```python
from build123d import *

# Parameters (mm, degrees)
PAD_DEPTH       = 9
SKETCH001_R     = 1.5
POCKET_DEPTH    = 13.501
SKETCH002_R     = 3
POCKET001_DEPTH = 11
PAD001_DEPTH    = 2
POCKET002_DEPTH = 2.501


with BuildPart() as part:
    # Sketch → Pad (new body)
    with BuildSketch(Plane.XY):
        with BuildLine():
            Line((-7, -4), (-31, -4))
            Line((-31, -4), (-31, -6.5))
            Line((-31, -6.5), (16, -6.5))
            Line((16, -6.5), (16, -3.5))
            Line((16, -3.5), (1.936492, -3.5))
            ThreePointArc((1.936492, 3.5), (-4, 0), (1.936492, -3.5))
            Line((1.936492, 3.5), (16, 3.5))
            Line((16, 7), (16, 3.5))
            Line((0, 7), (16, 7))
            Line((-7, 7), (0, 7))
            Line((-7, -4), (-7, 7))
        make_face()
    extrude(amount=PAD_DEPTH)

    # Sketch001 → Pocket (cut, through all)
    with BuildSketch(Plane.XZ.offset(6.5)):
        with Locations((-27.5, 4.5)):
            Circle(SKETCH001_R)
        with Locations((-8.5, 4.5)):
            Circle(SKETCH001_R)
        with Locations((10.5, 4.5)):
            Circle(SKETCH001_R)
    extrude(amount=-POCKET_DEPTH, mode=Mode.SUBTRACT)

    # Sketch002 → Pocket001 (cut)
    with BuildSketch(Plane(origin=(0, 7, 0), x_dir=(-1, 0, 0), z_dir=(0, 1, 0))):
        with Locations((8.5, 4.5)):
            Circle(SKETCH002_R)
    extrude(amount=-POCKET001_DEPTH, mode=Mode.SUBTRACT)

    # Sketch003 → Pad001 (new body)
    with BuildSketch(Plane(origin=(0, 7, 0), x_dir=(-1, 0, 0), z_dir=(0, 1, 0))):
        Polygon((-13.098076, 9), (-15.696152, 4.5), (-13.098076, 0), (-7.901924, 0), (-5.303848, 4.5), (-7.901924, 9), align=None)
        Polygon((-9, 1.901924), (-7.5, 4.5), (-9, 7.098076), (-12, 7.098076), (-13.5, 4.5), (-12, 1.901924), align=None, mode=Mode.SUBTRACT)
    extrude(amount=PAD001_DEPTH)

    # Sketch004 → Pocket002 (cut, through all)
    with BuildSketch(Plane(origin=(0, -4, 0), x_dir=(-1, 0, 0), z_dir=(0, 1, 0))):
        Polygon((31, 6), (28, 9), (31, 9), align=None)
        Polygon((28, 0), (31, 0), (31, 3), align=None)
    extrude(amount=-POCKET002_DEPTH, mode=Mode.SUBTRACT)


solid = part.part
```
Work out the finished part from the listing and answer in its coordinate system (mm). A direction names the side the tool comes from. Give positions to 0.01 mm unless a question says otherwise; leave off trailing zeros. Write each loop counter-clockwise with the first axis right and the second up, starting at its lowest first coordinate (ties: lowest second). Pieces come first, ordered by that corner, then holes. Notation, with made-up numbers: (50.25, -5.75) -> (91.25, -5.75) arc R32 ccw to (91.25, 31.25) -> close; hole circle Ø10 at (63, -17). An arc over 180 degrees is marked (long way). Write item = value, one per line.
Q1. Section B-B on x = 0 is taken. Determine the outline of the cut face in (y, z), and give its area (3 significant figures).
Computed values:
outline = (-6.5, 0) -> (-4, 0) -> (-4, 9) -> (-6.5, 9) -> close; (4, 0) -> (7, 0) -> (7, 9) -> (4, 9) -> close
area = 49.5 mm^2
Q2. A tool of negligible diameter and unlimited length cuts with its end or side. For faces 5 (the flat face through (14.415, 7.986, 2.281)), 6 (the flat face through (6.62, 7.99, 2.22)), 7 (the flat face through (-7, 1, 1)), 8 (the flat face through (8.24, 7.99, 5.78)), 9 (the flat face through (15.5, 7, 3.4)), from which of +Z, -Z, +X, -X, +Y, -Y can it reach the whole face along a straight path? Write none if from no direction.
Computed values:
face_5 = -Z, +X, +Y
face_6 = -Z, -X, +Y
face_7 = +Z, -Z, -X, +Y
face_8 = +Y
face_9 = +X, +Y
Q3. For a pull along Z with two mould halves and no side action, classify faces 1 (the flat face through (-7, 1, 8)), 2 (the flat face through (6.585, 7.986, 6.719)), 3 (the flat face through (11, 8, 1.902)), 4 (the cylindrical face through (9, -5.02, 4.57)) as pulls with the +Z half, pulls with the -Z half, needs draft (parallel to the pull), parting line crosses it, or undercut.
Computed values:
face_1 = needs draft
face_2 = pulls with the +Z half
face_3 = undercut
face_4 = undercut
Q4. Section A-A on x = 10.5 is taken. Determine the outline of the cut face in (y, z), and give its area (3 significant figures).
Computed values:
outline = (-6.5, 0) -> (-3.5, 0) -> (-3.5, 3) -> (-6.5, 3) -> close; (-6.5, 6) -> (-3.5, 6) -> (-3.5, 9) -> (-6.5, 9) -> close; (3.5, 0) -> (9, 0) -> (9, 1.9) -> (7, 1.9) -> (7, 3) -> (3.5, 3) -> close; (3.5, 6) -> (7, 6) -> (7, 7.1) -> (9, 7.1) -> (9, 9) -> (3.5, 9) -> close
area = 46.6 mm^2
Q5. Section C-C on z = 4 is taken. State how many separate pieces and enclosed holes the cut face has, and give its area (3 significant figures).
Computed values:
separate_pieces = 5
enclosed_holes = 0
area = 192 mm^2
Q6. Section D-D on y = 0 is taken. Determine the outline of the cut face in (x, z), and give its area (3 significant figures).
Computed values:
outline = (-7, 0) -> (-4, 0) -> (-4, 9) -> (-7, 9) -> (-7, 7.1) arc R3 cw to (-7, 1.9) -> close
area = 21.5 mm^2
Q7. Consider line 1 along Z through (x, y) = (-27.5, -5.05); line 2 along Y through (x, z) = (5, 7.25); line 3 along Y through (x, z) = (10, 7.75). Determine where each line is inside the solid, lowest interval first.
Computed values:
line_1 = 0 to 3, 6 to 9
line_2 = -6.5 to -3.5, 3.5 to 7
line_3 = -6.5 to -3.5, 3.5 to 9
Q8. Flat-ended cylindrical pins translate along their axes: pin 1 Ø1.5 at (x, z) = (-0.5, 7) entering from +Y; pin 2 Ø0.6 at (y, z) = (1, 8) entering from -X; pin 3 Ø4.5 at (x, z) = (-22, 4) entering from +Y. Find the tip coordinate at first contact, or state that the pin passes through.
Computed values:
pin_1 = 7
pin_2 = -7
pin_3 = -4
